from build123d import *

# Parameters (mm, degrees)
F0_W           = 249.260224402
F0_H           = 101.0710969567
F1_DEPTH       = 25.4
F3_D           = 7.1374
F3_CSINK_D     = 13.4874
F3_CSINK_ANGLE = 82
F4_D           = 7.1374
F4_CSINK_D     = 13.4874
F4_CSINK_ANGLE = 82


with BuildPart() as f1:
    # F0 (on Front) → F1 (new body)
    with BuildSketch(Plane.XZ):
        with Locations((-1.5978179872, -13.5989002883)):
            Rectangle(F0_W, F0_H)
    extrude(amount=-F1_DEPTH)

    # F3 (through all)
    with Locations(Plane.XZ):
        with Locations((-81.7563086748, -5.4461751133)):
            CounterSinkHole(F3_D / 2, F3_CSINK_D / 2, counter_sink_angle=F3_CSINK_ANGLE)

    # F4 (through all)
    with Locations(Plane.XZ):
        with Locations((11.5190250799, -8.2076163962), (83.6233198643, -11.2758828327)):
            CounterSinkHole(F4_D / 2, F4_CSINK_D / 2, counter_sink_angle=F4_CSINK_ANGLE)


solid = f1.part
Check sheet for the modelled part. Datum: model origin and axes. Units: mm. Give positions to 0.01 mm unless a question says otherwise; leave off trailing zeros. Return JSON: item names as keys, results as strings. Group by question number.
1. Mould release check, pull along Z, two halves, no side actions. Record for faces 1 (the flat face through (-3, 13, -64.134)), 2 (the cylindrical face through (80.327, 14.678, -12.643)), 3 (the flat face through (-3, 13, 36.937)): released by +Z, released by -Z, zero draft, split by the parting line, or undercut.
2. Go/stop test with flat-tipped pins: pin 1 (11.5 mm diameter, centred on x = 83.62, z = -11.28, fed in from -Y); pin 2 (12 mm diameter, centred on x = 92, z = -22.5, fed in from -Y). Record where each tip stops, or that it passes through.
3. Thickness scan on L1, parallel to X at y = 10, z = -11; L2, parallel to Z at x = 13, y = 19; L3, parallel to X at y = 17.5, z = -14. Record the ranges inside material, lowest first.
Return value:
{
 "1": {"face 1": "released by -Z", "face 2": "undercut", "face 3": "released by +Z"},
 "2": {"pin 1": "y = 1.14", "pin 2": "y = 0"},
 "3": {"L1": "-126.23 to 9.3, 13.74 to 80.07, 87.18 to 123.03", "L2": "-64.13 to -11.45, -4.96 to 36.94", "L3": "-126.23 to 81.32, 85.93 to 123.03"}
}
